Can you work these out from the model? Positions are in its coordinate system, mm. A direction names the side the tool comes from. Round coordinates to 2 decimals unless told otherwise and drop trailing zeros. Loops run counter-clockwise (first coordinate to the right, second up) from the corner with the lowest first, then second, coordinate; pieces in that order, holes last. Notation, with made-up numbers: (8, 2) -> (45, 2) arc R20 ccw to (45, 10) -> close; hole circle Ø3 at (46, 28.25). An arc over 180 degrees is marked (long way). Answer as a JSON object with one key per item and string values.
```python
from build123d import *

# Parameters (mm, degrees)
SKETCH1_R           = 15
BOSS_EXTRUDE1_DEPTH = 30
SKETCH2_R           = 7.5
CUT_EXTRUDE1_DEPTH  = 60
SKETCH3_W           = 15
SKETCH3_H           = 32
CUT_EXTRUDE2_DEPTH  = 101.543522914
RIB1_REACH          = 102.544
SKETCH4_WALL_W      = 281.406902826
SKETCH4_WALL_H      = 10


with BuildPart() as part:
    # Sketch1 → Boss-Extrude1 (new, symmetric)
    with BuildSketch(Plane.XY):
        with BuildLine():
            Line((30, 0), (30, -65))
            Line((30, -65), (53, -65))
            Line((53, -65), (53, -75))
            Line((53, -75), (33, -75))
            Line((33, -75), (33, -80))
            Line((33, -80), (20, -80))
            Line((20, -80), (10.9437787, -28))
            Line((10.9437787, -28), (-13.0562213, -28))
            Line((-13.0562213, -28), (-20, -80))
            Line((-20, -80), (-33, -80))
            Line((-33, -80), (-33, -75))
            Line((-33, -75), (-53, -75))
            Line((-53, -75), (-53, -65))
            Line((-53, -65), (-30, -65))
            Line((-30, -65), (-30, 0))
            ThreePointArc((-30, 0), (0, 30), (30, 0))
        make_face()
        Circle(SKETCH1_R, mode=Mode.SUBTRACT)
    extrude(amount=BOSS_EXTRUDE1_DEPTH, both=True)

    # Sketch2 → Cut-Extrude1 (cut)
    with BuildSketch(Plane(origin=(0, -65, 0), x_dir=(1, 0, 0), z_dir=(0, 1, 0))):
        with Locations(Location((41.5, 17.538074841, 0), (0, 0, 270))):
            Circle(SKETCH2_R)
        with Locations((41.5, -17.538074841)):
            Circle(SKETCH2_R)
    cut_extrude1 = extrude(amount=-CUT_EXTRUDE1_DEPTH, mode=Mode.SUBTRACT)

    # Mirror1: Cut-Extrude1 across plane
    add(cut_extrude1.mirror(Plane(origin=(0, 0, 0), x_dir=(0, 0, 1), z_dir=(1, 0, 0))), mode=Mode.SUBTRACT)

    # Sketch3 → Cut-Extrude2 (cut, through all)
    with BuildSketch(Plane(origin=(0, 0, 0), x_dir=(1, 0, 0), z_dir=(0, 1, 0))):
        Rectangle(SKETCH3_W, SKETCH3_H)
    extrude(amount=CUT_EXTRUDE2_DEPTH, mode=Mode.SUBTRACT)

    # Sketch4 wall → Rib1 (add, up to next)
    with BuildSketch(Plane(origin=(-40.746781429, -27.806470527, 0), x_dir=(-0.312901964861, -0.949785428603, 0), z_dir=(0.949785428603, -0.312901964861, 0)), mode=Mode.PRIVATE) as rib1_sk1:
        Rectangle(SKETCH4_WALL_W, SKETCH4_WALL_H)
    rib1_tool1 = extrude(rib1_sk1.sketch, amount=RIB1_REACH, mode=Mode.PRIVATE) - part.part
    rib1 = rib1_tool1.solids().sort_by_distance((-40.746781429, -27.806470527, 0))[0]
    add(rib1)

    # Mirror2: Rib1 across plane
    add(rib1.mirror(Plane(origin=(0, 0, 0), x_dir=(0, 0, 1), z_dir=(1, 0, 0))))


solid = part.part
```
Q1. I want a section at C-C, the plane z = 1.5. Write out the boundary of the cut face in (x, y), then the cut area to 3 significant figures.
Determined:
{"outline": "(-53, -75) -> (-33, -75) -> (-33, -80) -> (-20, -80) -> (-13.06, -28) -> (10.94, -28) -> (20, -80) -> (33, -80) -> (33, -75) -> (53, -75) -> (53, -65) -> (28.49, 9.39) arc R30 ccw to (7.5, 29.05) -> (7.5, 12.99) arc R15 cw (long way) to (-7.5, 12.99) -> (-7.5, 29.05) arc R30 ccw to (-28.49, 9.39) -> (-53, -65) -> close", "area": "5,710 mm²"}
Q2. If I drill on L1, parallel to Z at x = -41, y = -67; L2, parallel to Z at x = -41.5, y = -68; L3, parallel to Y at x = 0, z = -15.5, over which ranges is the centre line in solid material (lowest first)? Write a range as [from, to].
Determined:
{"L1": "[-30, -25.02], [-10.05, 10.05], [25.02, 30]", "L2": "[-30, -25.04], [-10.04, 10.04], [25.04, 30]", "L3": "[-28, -15]"}
Q3. I want a section at A-A, the plane y = -68. Write out the boundary of the cut face in (x, z).
Determined:
{"outline": "(-53, -30) -> (-18.4, -30) -> (-18.4, 30) -> (-53, 30) -> close; (17.91, -30) -> (53, -30) -> (53, 30) -> (17.91, 30) -> close; hole circle Ø15 at (-41.5, -17.54); hole circle Ø15 at (-41.5, 17.54); hole circle Ø15 at (41.5, -17.54); hole circle Ø15 at (41.5, 17.54)"}
Q4. I want a section at B-B, the plane x = 0. Write out the boundary of the cut face in (y, z).
Determined:
{"outline": "(-28, -30) -> (-15, -30) -> (-15, 30) -> (-28, 30) -> close; (15, -30) -> (30, -30) -> (30, -16) -> (15, -16) -> close; (15, 16) -> (30, 16) -> (30, 30) -> (15, 30) -> close"}
Q5. I'm going to push flat-ended pins straight in: pin 1 (1 mm diameter, centred on y = -25.5, z = 3.5, fed in from -X); pin 2 (8 mm diameter, centred on y = 24.5, z = 7.5, fed in from -X); pin 3 (17 mm diameter, centred on x = 41.5, z = -17.54, fed in from +Y). Where does each tip first touch, or does it pass through?
Determined:
{"pin 1": "x = -40.15", "pin 2": "x = -21.9", "pin 3": "y = -65"}
Q6. On a 3-axis mill with a long thin cutter (end or side, diameter ignored), from which of +Z, -Z, +X, -X, +Y, -Y can I reach the whole of each face in a straight line? I mean faces 4 (the flat face through (43, -75, 0)), 5 (the flat face through (-47, -65, 23)), 6 (the flat face through (7.5, 21, 0)), 7 (the flat face through (15.535, -54.364, 0.42)), 8 (the flat face through (40, -46, 5)). Say none if no direction works.
Determined:
{"face 4": "+Z, -Z, +X, -Y", "face 5": "+Z, -X, +Y", "face 6": "+Y", "face 7": "+Z, -Z, -Y", "face 8": "+Z, +X, +Y"}
Q7. We'd pull the mould along X, two halves only. Please class faces 1 (the flat face through (-30, -33, 18)), 2 (the cylindrical face through (40.524, -69.93, 10.102)), 3 (the flat face through (1, -24, 30)): pulls with the +X half, pulls with the -X half, needs draft (parallel to the pull), parting line crosses it, or undercut.
Determined:
{"face 1": "pulls with the -X half", "face 2": "undercut", "face 3": "needs draft"}
Q8. I want a section at D-D, the plane y = -33. Write out the boundary of the cut face in (x, z).
Determined:
{"outline": "(-42.46, -5) -> (-30, -5) -> (-30, -30) -> (-13.72, -30) -> (-13.72, 30) -> (-30, 30) -> (-30, 5) -> (-42.46, 5) -> close; (11.81, -30) -> (30, -30) -> (30, -5) -> (42.46, -5) -> (42.46, 5) -> (30, 5) -> (30, 30) -> (11.81, 30) -> close"}
